```python
from build123d import *

# Parameters (mm, degrees)
SKETCH1_R           = 6.35
BOSS_EXTRUDE1_DEPTH = 7.62
SKETCH2_W           = 2.54
SKETCH2_H           = 2.54
BOSS_EXTRUDE2_DEPTH = 5.08
SKETCH3_R           = 3.048
CUT_EXTRUDE1_DEPTH  = 3.81


with BuildPart() as part:
    # Sketch1 → Boss-Extrude1 (new body)
    with BuildSketch(Plane.XY):
        with Locations(Location((0, 0, 0), (0, 0, 180))):
            Circle(SKETCH1_R)
    extrude(amount=BOSS_EXTRUDE1_DEPTH)

    # Sketch2 → Boss-Extrude2 (add)
    with BuildSketch(Plane.XY.offset(7.62)):
        with BuildLine():
            Line((-1.27, 1.27), (1.27, 1.27))
            Line((1.27, 1.27), (1.27, 6.221703947))
            ThreePointArc((1.27, 6.221703947), (0, 6.35), (-1.27, 6.221703947))
            Line((-1.27, 6.221703947), (-1.27, 1.27))
        make_face()
        with BuildLine():
            Line((-6.221703947, -1.27), (-1.27, -1.27))
            Line((-1.27, -1.27), (-1.27, 1.27))
            Line((-1.27, 1.27), (-6.221703947, 1.27))
            ThreePointArc((-6.221703947, 1.27), (-6.35, 0), (-6.221703947, -1.27))
        make_face()
        Rectangle(SKETCH2_W, SKETCH2_H)
        with BuildLine():
            Line((1.27, 1.27), (1.27, -1.27))
            Line((1.27, -1.27), (6.221703947, -1.27))
            ThreePointArc((6.221703947, -1.27), (6.317844572, -0.638231909), (6.35, 0))
            ThreePointArc((6.35, 0), (6.317844572, 0.638231909), (6.221703947, 1.27))
            Line((6.221703947, 1.27), (1.27, 1.27))
        make_face()
        with BuildLine():
            ThreePointArc((-1.27, -6.221703947), (0, -6.35), (1.27, -6.221703947))
            Line((1.27, -6.221703947), (1.27, -1.27))
            Line((1.27, -1.27), (-1.27, -1.27))
            Line((-1.27, -1.27), (-1.27, -6.221703947))
        make_face()
    extrude(amount=BOSS_EXTRUDE2_DEPTH)

    # Sketch3 → Cut-Extrude1 (cut)
    with BuildSketch(Plane(origin=(0, 0, 0), x_dir=(-1, 0, 0), z_dir=(0, 0, -1))):
        Circle(SKETCH3_R)
    extrude(amount=-CUT_EXTRUDE1_DEPTH, mode=Mode.SUBTRACT)


solid = part.part
```
Verification items for the finished model (mm, model axes). A direction names the side the tool comes from. Coordinates: 2 decimals unless noted, no trailing zeros. Loops run counter-clockwise (first coordinate to the right, second up) from the corner with the lowest first, then second, coordinate; pieces in that order, holes last. Notation, with made-up numbers: (15, 37) - (59, 37) arc R30 cw to (59, 61) - close; hole circle Ø10 at (23, 12). An arc over 180 degrees is marked (long way). Put each result on its own line as item: value.
Item 1: Section check D-D (x = -2.25). Enter the section's corners in (y, z), then the cut area to 3 significant figures.
Conclusion:
outline: (-5.94, 0) - (-2.06, 0) - (-2.06, 3.81) - (2.06, 3.81) - (2.06, 0) - (5.94, 0) - (5.94, 7.62) - (1.27, 7.62) - (1.27, 12.7) - (-1.27, 12.7) - (-1.27, 7.62) - (-5.94, 7.62) - close
area: 87.7 mm2
Item 2: Gauge pin test, flat ends, axial feed: pin 1 Ø3 at (y, z) = (2, 3) entering from +X; pin 2 Ø1.5 at (y, z) = (-5, 2) entering from +X; pin 3 Ø2.5 at (x, z) = (-3.5, 10.5) entering from -Y. Record the tip position at first contact, or that the pin passes through.
Conclusion:
pin 1: stops at x = 6.33
pin 2: stops at x = 4.72
pin 3: stops at y = -1.27
Item 3: Section check A-A (z = 11.25). Enter the section's corners in (x, y), then the cut area to 3 significant figures.
Conclusion:
outline: (-6.22, -1.27) - (-1.27, -1.27) - (-1.27, -6.22) arc R6.35 ccw to (1.27, -6.22) - (1.27, -1.27) - (6.22, -1.27) arc R6.35 ccw to (6.22, 1.27) - (1.27, 1.27) - (1.27, 6.22) arc R6.35 ccw to (-1.27, 6.22) - (-1.27, 1.27) - (-6.22, 1.27) arc R6.35 ccw to start
area: 57.6 mm2
Item 4: Set-up check for faces 1 (the face through (1.27, 4, 10)), 2 (the face through (3, -3, 7.62)), 3 (the face through (-4, -1.27, 10)), 4 (the face through (-1.27, 4, 10)): record each of +Z, -Z, +X, -X, +Y, -Y from which the full face is reachable in a straight line by a thin tool's end or side.
Conclusion:
face 1: +Z, +X, +Y
face 2: +Z, +X, -Y
face 3: +Z, -X, -Y
face 4: +Z, -X, +Y
Item 5: Section check C-C (z = 2.5). Enter the section's corners in (x, y).
Conclusion:
outline: circle Ø12.7 at (0, 0); hole circle Ø6.1 at (0, 0)
Item 6: Draft check along X on faces 5 (the face through (1.27, -4, 10)), 6 (the face through (0, 0, 3.81)), 7 (the face through (-3, -3, 7.62)), 8 (the face through (0.4, 3.02, 1.88)). Enter one of: pulls with the +X half, pulls with the -X half, needs draft (parallel to the pull), parting line crosses it, or undercut.
Conclusion:
face 5: pulls with the +X half
face 6: undercut
face 7: needs draft
face 8: undercut
Item 7: Scan lines: line 1 along Y through (x, z) = (0, 1.05); line 2 along Y through (x, z) = (3.75, 8). Record each from-to range of solid material in increasing order.
Conclusion:
line 1: y = -6.35 to -3.05, 3.05 to 6.35
line 2: y = -1.27 to 1.27
Item 8: Section check B-B (y = 0). Enter the section's corners in (x, z), then the cut area to 3 significant figures.
Conclusion:
outline: (-6.35, 0) - (-3.05, 0) - (-3.05, 3.81) - (3.05, 3.81) - (3.05, 0) - (6.35, 0) - (6.35, 12.7) - (-6.35, 12.7) - close
area: 138 mm2
